Autodesk Inventor part; units mm, degrees
ref_plane "YZ Plane" through (0, 0, 0) normal (1, 0, 0) x (0, 1, 0)
ref_plane "XZ Plane" through (0, 0, 0) normal (0, 1, 0) x (-1, 0, 0)
ref_plane "XY Plane" through (0, 0, 0) normal (0, 0, 1) x (1, 0, 0)
sketch "Sketch1" plane through (0, 0, 0) normal (0, 0, 1) x (1, 0, 0)
  arc A0 (-6, 0) -> (6, 0) centre (0, 0) ccw
  arc A1 (0, -8) -> (8, 0) centre (0, 0) ccw
  line L0 (-6, -14) -> (-6, -50)
  line L1 (-8, 0) -> (-8, -50)
  line L2 (-6, 0) -> (-6, 20)
  line L3 (-8, 0) -> (-8, 20)
  line L4 (6, 0) -> (6, 20)
  line L5 (8, 0) -> (8, 20)
  line L6 (-8, -50) -> (-6, -50)
  line L7 (26.4346, -8) -> (-30.23, -8) construction
  arc A2 (0, -8) -> (-6, -14) centre (0, -14) ccw
  line L8 (8, 20) -> (6, 20)
  line L9 (-6, 20) -> (-8, 20)
  arc A3 (6, 0) -> (-6, 0) centre (0, 0) ccw construction
  dimension "d0" = 12
  dimension "d1" = 2
  dimension "d2" = 42
  dimension "d3" = 20
  dimension "d4" = 20
extrude "Extrusion1" add sketch "Sketch1" along normal blind 14
sketch "Sketch3" plane through (-8, -50, 0) normal (-1, 0, 0) x (0, 0, 1)
  line L0 (0, 0) -> (0, 70)
  line L1 (0, 0) -> (14, 0)
  line L2 (14, 70) -> (14, 0)
  line L3 (0, 70) -> (14, 70)
  line L4 (0, 42) -> (14, 42)
  circle A0 centre (6, 24.5) radius 1.5
  circle A1 centre (6, 5.5) radius 1.5
  line L5 (10.141, 23) -> (1.2635, 23) construction
  line L6 (10.6037, 7) -> (1.7262, 7) construction
  line L7 (6, 3.0673) -> (6, 29.9023) construction
  line L8 (9.9327, 26) -> (0.2455, 26) construction
  line L9 (10.6205, 4) -> (2.6453, 4) construction
  circle A2 centre (7, 63) radius 2
  line L10 (14, 54) -> (0, 54) construction
  point P0 (0, 50)
  dimension "d7" = 3
  dimension "d8" = 3
  dimension "d9" = 16
  dimension "d10" = 22
  dimension "d11" = 4
  dimension "d12" = 14
  dimension "d13" = 6
  dimension "d14" = 4
  dimension "d15" = 7
  dimension "d16" = 7
  dimension "d17" = 12
extrude "Extrusion2" cut sketch "Sketch3" against normal up to surface (16 mm away) contours A0 | A1 | A2
fillet "Fillet1" radius 1 17 edges at (8, 20, 7) (6, 20, 7) (-6, 20, 7) (-8, 20, 7) (-6, -50, 7) (-8, -50, 7) (-4.2426, -9.7574, 14) (5.6569, -5.6569, 14) (8, 10, 14) (-6, -32, 14) (-6, 10, 14) (6, 10, 14) (0, -6, 14) (-8, -15, 14) (-7, -50, 14) (7, 20, 14) (-7, 20, 14)
equation "\"d8\" = d7"
equation "\"d16\" = 0.5 * d12"
properties part number "Ø12-Z Endstop Holder"
Source: CAD feature listing. Evaluate the final solid. Frame: model axes, mm. A direction names the side the tool comes from. Round coordinates to 2 decimals unless told otherwise and drop trailing zeros. Answer as a JSON object with one key per item and string values. Group by question number.
(1) Reachability of faces 1 (the flat face through (6, 9, 6)), 2 (the flat face through (8, 9, 6)), 3 (the flat face through (-6, -31, 6)) from +Z, -Z, +X, -X, +Y, -Y: full face, straight path, thin tool, end or side. Return the list, or none.
(2) Mould query, pull axis X, two halves, no side actions, for faces 4 (the cylindrical face through (-7, -46, 6)), 5 (the cylindrical face through (5.719, -5.594, 6.409)), 6 (the flat face through (-8, -15, 6)), 7 (the flat face through (-6, 9, 6)). Classes: +X half, -X half, draft (parallel to the pull), parting line (faces both ways), or undercut.
(3) First-contact query: pin 1 (5 mm diameter, centred on x = -4.5, y = -26, fed in from +Z); pin 2 (2.5 mm diameter, centred on y = 13, z = 7, fed in from -X); pin 3 (4 mm diameter, centred on y = -38.5, z = 12.5, fed in from +X); pin 4 (3 mm diameter, centred on y = -2, z = 9.5, fed in from +X). Flat tips, straight axial feed; report the tip coordinate or a pass-through.
(4) Section query C-C on z = 6. State how many separate pieces and enclosed holes the cut face has, then the cut area to 3 significant figures.
(5) Ray query, line 1 (X direction, y = 13.5, z = 1); line 2 (Y direction, x = -6.95, z = 6); line 3 (Y direction, x = -6.65, z = 6). Return the intervals inside material, ascending. Write a range as [from, to].
Computed values:
{
 "1": {"face 1": "+Z, -Z, +Y", "face 2": "+Z, -Z, +X, +Y, -Y", "face 3": "+Z, -Z, +X, -Y"},
 "2": {"face 4": "draft", "face 5": "+X half", "face 6": "-X half", "face 7": "undercut"},
 "3": {"pin 1": "z = 14", "pin 2": "through", "pin 3": "x = -6", "pin 4": "x = 7.98"},
 "4": {"separate pieces": "5", "enclosed holes": "0", "area": "202 mm^2"},
 "5": {"line 1": "[-8, -6], [6, 8]", "line 2": "[-50, -46], [-43, -27], [-24, 11.27], [14.73, 20]", "line 3": "[-49.94, -46], [-43, -27], [-24, 11.27], [14.73, 19.94]"}
}
